Answer from the drawing. Dimensions are ordinates in mm from the lowest x, y and z of the part. A direction names the side the tool comes from. Give positions to 0.01 mm unless a question says otherwise; leave off trailing zeros. Loops run counter-clockwise (first coordinate to the right, second up) from the corner with the lowest first, then second, coordinate; pieces in that order, holes last.
(1) Which of the six approach directions +Z, -Z, +X, -X, +Y, -Y give full straight-line access (tool end or side, diameter ignored) to the marked faces 1, 2 and 3?
(2) Find section A-A, the plane x = 35. Write down the section's boundary in (y, z), then the cut area to 3 significant figures.
(3) Straight lines are drawn through the part: probe 1 along Y at (x, z) = (3, 0.95); probe 2 along Z at (x, y) = (17, 10.75); probe 3 along Y at (x, z) = (31, 8.75). For each, find the intervals that lie inside material, in ascending order.
(4) Find section C-C, the plane x = 3. Write down the section's boundary in (y, z).
(5) Each of these flat-tipped pins is pushed along its axis until it touches: P1, Ø3.5, axis at x = 32, z = 6.5, coming from the -Y side; P2, Ø1, axis at x = 26.5, z = 1, coming from the -Y side; P3, Ø1.6, axis at y = 5, z = 0.5, coming from the +X side. Where does it stop, or does it pass through?
(6) Find section D-D, the plane z = 1. Write down the section's boundary in (x, y), then the cut area to 3 significant figures.
(7) Find section B-B, the plane y = 3. Write down the section's boundary in (x, z), then the cut area to 3 significant figures.
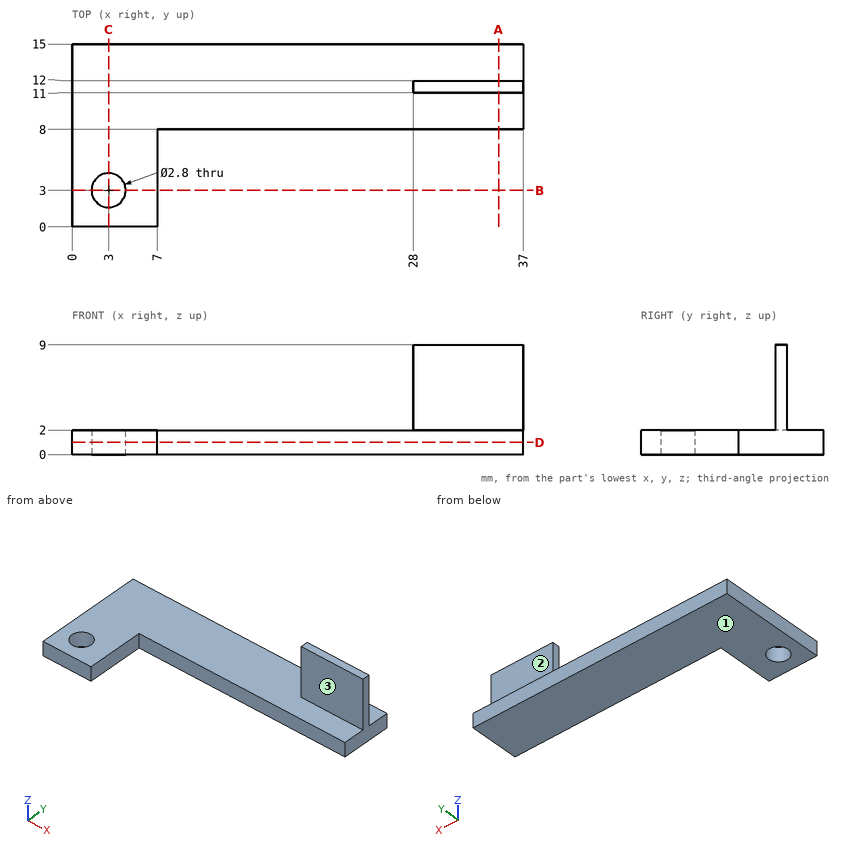
Entries:
1. face 1: -Z, +X, -X, +Y, -Y
1. face 2: +Z, +X, -X, +Y
1. face 3: +Z, +X, -X, -Y
2. outline: (8, 0) - (15, 0) - (15, 2) - (12, 2) - (12, 9) - (11, 9) - (11, 2) - (8, 2) - close
2. area: 21.0 mm2
3. probe 1: y = 0 to 1.6, 4.4 to 15
3. probe 2: z = 0 to 2
3. probe 3: y = 11 to 12
4. outline: (0, 0) - (1.6, 0) - (1.6, 2) - (0, 2) - close; (4.4, 0) - (15, 0) - (15, 2) - (4.4, 2) - close
5. P1: stops at y = 11
5. P2: stops at y = 8
5. P3: stops at x = 7
6. outline: (0, 0) - (7, 0) - (7, 8) - (37, 8) - (37, 15) - (0, 15) - close; hole circle Ø2.8 at (3, 3)
6. area: 309 mm2
7. outline: (0, 0) - (1.6, 0) - (1.6, 2) - (0, 2) - close; (4.4, 0) - (7, 0) - (7, 2) - (4.4, 2) - close
7. area: 8.40 mm2
